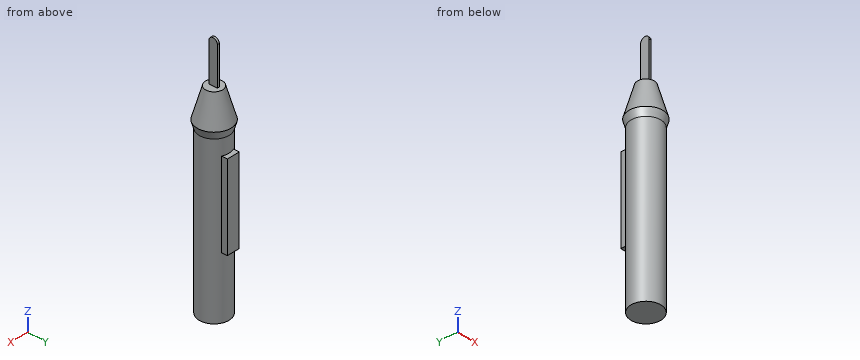
```python
from build123d import *

# Parameters (mm, degrees)
BOSS_EXTRUDE1_DEPTH = 0.5
SKETCH3_W           = 6
SKETCH3_H           = 40
BOSS_EXTRUDE2_DEPTH = 9


with BuildPart() as part:
    # Sketch1 → Boss-Extrude1 (new body, symmetric)
    with BuildSketch(Plane(origin=(0, 0, 0), x_dir=(0, 0, -1), z_dir=(1, 0, 0))):
        with BuildLine():
            Line((2, 2), (20, 2))
            Line((20, 2), (20, -2))
            Line((20, -2), (2, -2))
            ThreePointArc((2, -2), (0, 0), (2, 2))
        make_face()
    extrude(amount=BOSS_EXTRUDE1_DEPTH, both=True)

    # Sketch2 → Revolve1 (revolve)
    with BuildSketch(Plane(origin=(0, 0, 0), x_dir=(0, 0, -1), z_dir=(1, 0, 0))):
        Polygon((20, 0), (20, 4), (34, 8), (37.495076137, 6.998076938), (114, 6.998076938), (114, 0), (34, 0), align=None)
    revolve(axis=Axis((0, 0, -20), (0, 0, -1)))

    # Sketch3 → Boss-Extrude2 (add)
    with BuildSketch(Plane(origin=(0, 0, 0), x_dir=(1, 0, 0), z_dir=(0, 1, 0))):
        with Locations((0, 64.847291261)):
            Rectangle(SKETCH3_W, SKETCH3_H)
    extrude(amount=BOSS_EXTRUDE2_DEPTH)


solid = part.part
```
Verification items for the finished model (mm, model axes). Coordinates: 2 decimals unless noted, no trailing zeros. Loops run counter-clockwise (first coordinate to the right, second up) from the corner with the lowest first, then second, coordinate; pieces in that order, holes last. Notation, with made-up numbers: (16.25, 76) - (30.25, 76) arc R19 ccw to (30.25, 87) - close; hole circle Ø9 at (59, 55.25). An arc over 180 degrees is marked (long way). Answer as a JSON object with one key per item and string values.
(1) Scan lines: line 1 along Z through (x, y) = (-1.75, 2); line 2 along X through (y, z) = (-0.75, -7); line 3 along Z through (x, y) = (-0.75, 8.5). Record each from-to range of solid material in increasing order.
Response:
{"line 1": "z = -114 to -20", "line 2": "x = -0.5 to 0.5", "line 3": "z = -84.85 to -44.85"}
(2) Cross-section at A-A, the plane y = 0. Record the boundary of the cut face in (x, z), then the cut area to 3 significant figures.
Response:
{"outline": "(-8, -34) - (-7, -37.5) - (-7, -114) - (7, -114) - (7, -37.5) - (8, -34) - (4, -20) - (0.5, -20) - (0.5, 0) - (-0.5, 0) - (-0.5, -20) - (-4, -20) - close", "area": "1,310 mm²"}
(3) Cross-section at B-B, the plane z = -46. Record the boundary of the cut face in (x, y).
Response:
{"outline": "(-3, 6.32) arc R7 ccw (long way) to (3, 6.32) - (3, 9) - (-3, 9) - close"}
(4) Go/stop test with flat-tipped pins: pin 1 Ø0.8 at (y, z) = (7.5, -61.5) entering from +X; pin 2 Ø3 at (y, z) = (7, -58.5) entering from -X; pin 3 Ø1.3 at (x, y) = (-0.5, 8) entering from -Z; pin 4 Ø4 at (x, y) = (-1.5, 1.5) entering from +Z. Record where each tip stops, or that it passes through.
Response:
{"pin 1": "stops at x = 3", "pin 2": "stops at x = -4.33", "pin 3": "stops at z = -84.85", "pin 4": "stops at z = 0"}
